For this review, use the dimensioned drawing (mm, ordinates from the lowest corner) and the shaded views. Give positions to 0.01 mm unless a question says otherwise; leave off trailing zeros. Order: outer loops, then holes, each group sorted by start corner. A loop starts at its lowest first (then second) coordinate and runs counter-clockwise, first axis right, second up. Notation, with made-up numbers: (12.5, -38.75) - (45.5, -38.75) arc R37 ccw to (45.5, -0.75) - close; hole circle Ø2 at (22, 24). An arc over 180 degrees is marked (long way). Use a Markdown table: item, result. Add a question column.
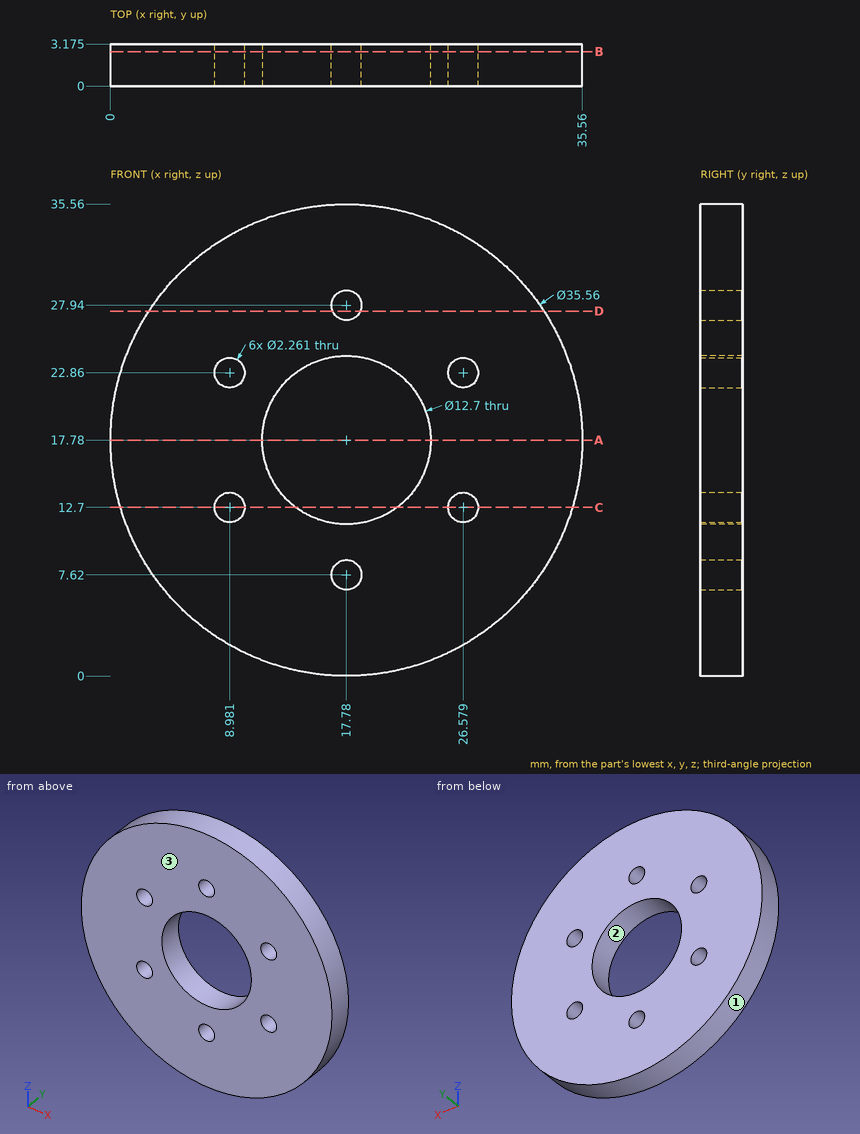
Q1. Wall thickness on probe 1 along Z at (x, y) = (17.78, 1.3); probe 2 along X at (y, z) = (2.5, 18); probe 3 along Z at (x, y) = (9.5, 2.85) (1 decimal): over which ranges is each line inside the solid? List them lowest first.
Q2. We need section D-D (z = 27.5). Write out the cut boundary in (x, y) (1 decimal).
Q3. We need section B-B (y = 2.6). Write out the cut boundary in (x, z).
Q4. We need section A-A (z = 17.78). Write out the cut boundary in (x, y) (1 decimal).
Q5. We need section C-C (z = 12.7). Write out the cut boundary in (x, y) (1 decimal).
Q6. Draft analysis for pull direction Z (two halves, no side actions). For the marked faces 1, 2 and 3, state which applies: pulls with the +Z half, pulls with the -Z half, needs draft (parallel to the pull), parting line crosses it, or undercut.
Here are the results:
| question | item | result |
|---|---|---|
| 1 | probe 1 | 0 to 6.49, 8.75 to 11.43, 24.13 to 26.81, 29.07 to 35.56 |
| 1 | probe 2 | 0 to 11.43, 24.13 to 35.56 |
| 1 | probe 3 | 2 to 11.7, 13.7 to 21.9, 23.9 to 33.5 |
| 2 | outline | (2.9, 0) - (16.7, 0) - (16.7, 3.2) - (2.9, 3.2) - close; (18.8, 0) - (32.7, 0) - (32.7, 3.2) - (18.8, 3.2) - close |
| 3 | outline | circle Ø35.56 at (17.78, 17.78); hole circle Ø2.26 at (8.98, 12.7); hole circle Ø2.26 at (8.98, 22.86); hole circle Ø12.7 at (17.78, 17.78); hole circle Ø2.26 at (17.78, 7.62); hole circle Ø2.26 at (17.78, 27.94); hole circle Ø2.26 at (26.58, 12.7); hole circle Ø2.26 at (26.58, 22.86) |
| 4 | outline | (0, 0) - (11.4, 0) - (11.4, 3.2) - (0, 3.2) - close; (24.1, 0) - (35.6, 0) - (35.6, 3.2) - (24.1, 3.2) - close |
| 5 | outline | (0.7, 0) - (7.9, 0) - (7.9, 3.2) - (0.7, 3.2) - close; (10.1, 0) - (14, 0) - (14, 3.2) - (10.1, 3.2) - close; (21.6, 0) - (25.4, 0) - (25.4, 3.2) - (21.6, 3.2) - close; (27.7, 0) - (34.8, 0) - (34.8, 3.2) - (27.7, 3.2) - close |
| 6 | face 1 | parting line crosses it |
| 6 | face 2 | undercut |
| 6 | face 3 | needs draft |
